Read the model definition and answer for the solid it produces. Units are mm, in the model's axes. Face numbers are marked on the shaded views. A direction names the side the tool comes from. Coordinates: 2 decimals unless noted, no trailing zeros. Write each loop counter-clockwise with the first axis right and the second up, starting at its lowest first coordinate (ties: lowest second). Pieces come first, ordered by that corner, then holes. Notation, with made-up numbers: (-8.75, 31.25) -> (29.25, 31.25) arc R8 ccw to (29.25, 41.25) -> close; hole circle Ø10 at (-7.5, 62). An arc over 180 degrees is marked (long way). Answer as a JSON object with one key per item and string values. Group by question number.
(1) Find section D-D (z = 3). Give the vertices of the cut face in (x, y).
(2) For a pull along X with two mould halves and no side action, classify the marked faces 3 and 4 as +X half, -X half, draft (parallel to the pull), parting line (faces both ways), or undercut.
(3) Which of the six approach directions +Z, -Z, +X, -X, +Y, -Y give full straight-line access (tool end or side, diameter ignored) to the marked faces 1 and 2?
(4) Find section A-A (x = 86). Give the vertices of the cut face in (y, z), then the cut area to 3 significant figures.
(5) Flat-ended cylindrical pins translate along their axes: P1, Ø16, axis at x = 86, y = 0, coming from the +Z side; P2, Ø2, axis at x = -27, z = 7, coming from the -Y side; P3, Ø10, axis at y = 7.5, z = 8.5, coming from the +X side; P4, Ø11.5, axis at x = 0, y = 0, coming from the -Z side. Find the tip coordinate at first contact, or state that the pin passes through.
(6) Find section B-B (y = 17). Give the vertices of the cut face in (x, z).
(7) Straight lines are drawn through the part: L1, parallel to Y at x = 86, z = 6.5; L2, parallel to Y at x = 0, z = 15.75; L3, parallel to X at y = 7, z = 19.5. For each, find the intervals that lie inside material, in ascending order.
(8) Find section C-C (x = 0). Give the vertices of the cut face in (y, z).
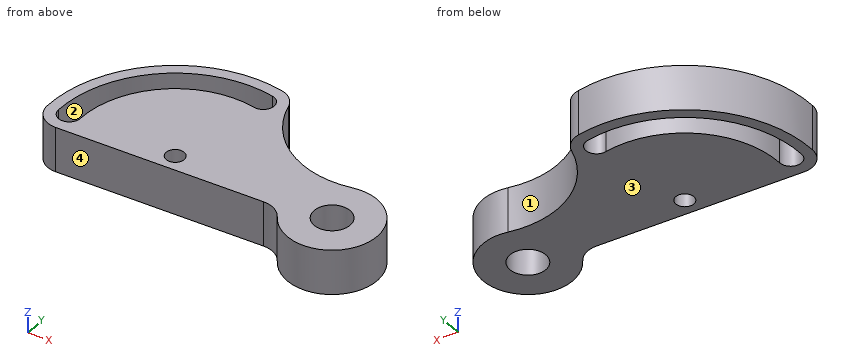
from build123d import *

# Parameters (mm, degrees)
F0_R     = 5
F0_R_2   = 10
F1_DEPTH = 25


with BuildPart() as f1:
    # F0 (on Top) → F1 (new body)
    with BuildSketch(Plane.XY):
        with BuildLine():
            ThreePointArc((53.104685, -7.013139), (59.758753, -8.503991), (64.74277, -13.157895))
            ThreePointArc((64.74277, -13.157895), (109.023376, -9.742904), (80.644633, 24.419665))
            ThreePointArc((80.644633, 24.419665), (43.979871, 30.522731), (21.657847, 60.242749))
            ThreePointArc((21.657847, 60.242749), (18.171776, 65.972496), (12.155372, 68.936543))
            ThreePointArc((12.155372, 68.936543), (-44.995133, 53.623111), (-70, 0))
            ThreePointArc((-70, 0), (-66.29239, -8.673884), (-57.460622, -11.987872))
            Line((-57.460622, -11.987872), (53.104685, -7.013139))
        make_face()
        Circle(F0_R, mode=Mode.SUBTRACT)
        with Locations((86, 0)):
            Circle(F0_R_2, mode=Mode.SUBTRACT)
        with BuildLine():
            ThreePointArc((-64, 0), (-41.138407, 49.026844), (11.113483, 63.027696))
            ThreePointArc((11.113483, 63.027696), (15.980441, 56.076961), (9.029705, 51.210003))
            ThreePointArc((9.029705, 51.210003), (-33.424956, 39.834311), (-52, 0))
            ThreePointArc((-52, 0), (-58, -6), (-64, 0))
        make_face(mode=Mode.SUBTRACT)
    extrude(amount=F1_DEPTH)


solid = f1.part
Results below:
{
 "1": {"outline": "(-70, 0) arc R12 ccw to (-57.46, -11.99) -> (53.1, -7.01) arc R13 cw to (64.74, -13.16) arc R25 ccw (long way) to (80.64, 24.42) arc R50 cw to (21.66, 60.24) arc R12 ccw to (12.16, 68.94) arc R70 ccw to start; hole (-64, 0) arc R6 ccw to (-52, 0) arc R52 cw to (9.03, 51.21) arc R6 ccw to (11.11, 63.03) arc R64 ccw to start; hole circle Ø10 at (0, 0); hole circle Ø20 at (86, 0)"},
 "2": {"face 3": "draft", "face 4": "undercut"},
 "3": {"face 1": "+Z, -Z, +Y", "face 2": "+Z, -Z"},
 "4": {"outline": "(-25, 0) -> (-10, 0) -> (-10, 25) -> (-25, 25) -> close; (10, 0) -> (25, 0) -> (25, 25) -> (10, 25) -> close", "area": "750 mm2"},
 "5": {"P1": "passes through", "P2": "stops at y = -10.66", "P3": "stops at x = 110.87", "P4": "stops at z = 0"},
 "6": {"outline": "(-67.9, 0) -> (-61.7, 0) -> (-61.7, 25) -> (-67.9, 25) -> close; (-49.14, 0) -> (104.33, 0) -> (104.33, 25) -> (-49.14, 25) -> close"},
 "7": {"L1": "y = -25 to -10, 10 to 25", "L2": "y = -9.4 to -5, 5 to 52, 64 to 70", "L3": "x = -69.65 to -63.62, -51.53 to 78.86, 93.14 to 110"},
 "8": {"outline": "(-9.4, 0) -> (-5, 0) -> (-5, 25) -> (-9.4, 25) -> close; (5, 0) -> (52, 0) -> (52, 25) -> (5, 25) -> close; (64, 0) -> (70, 0) -> (70, 25) -> (64, 25) -> close"}
}
